Part print with two shaded views. Sizes in mm from the minimum x, y, z corner. A direction names the side the tool comes from. Give positions to 0.01 mm unless a question says otherwise; leave off trailing zeros. Write each loop counter-clockwise with the first axis right and the second up, starting at its lowest first coordinate (ties: lowest second). Pieces come first, ordered by that corner, then holes.
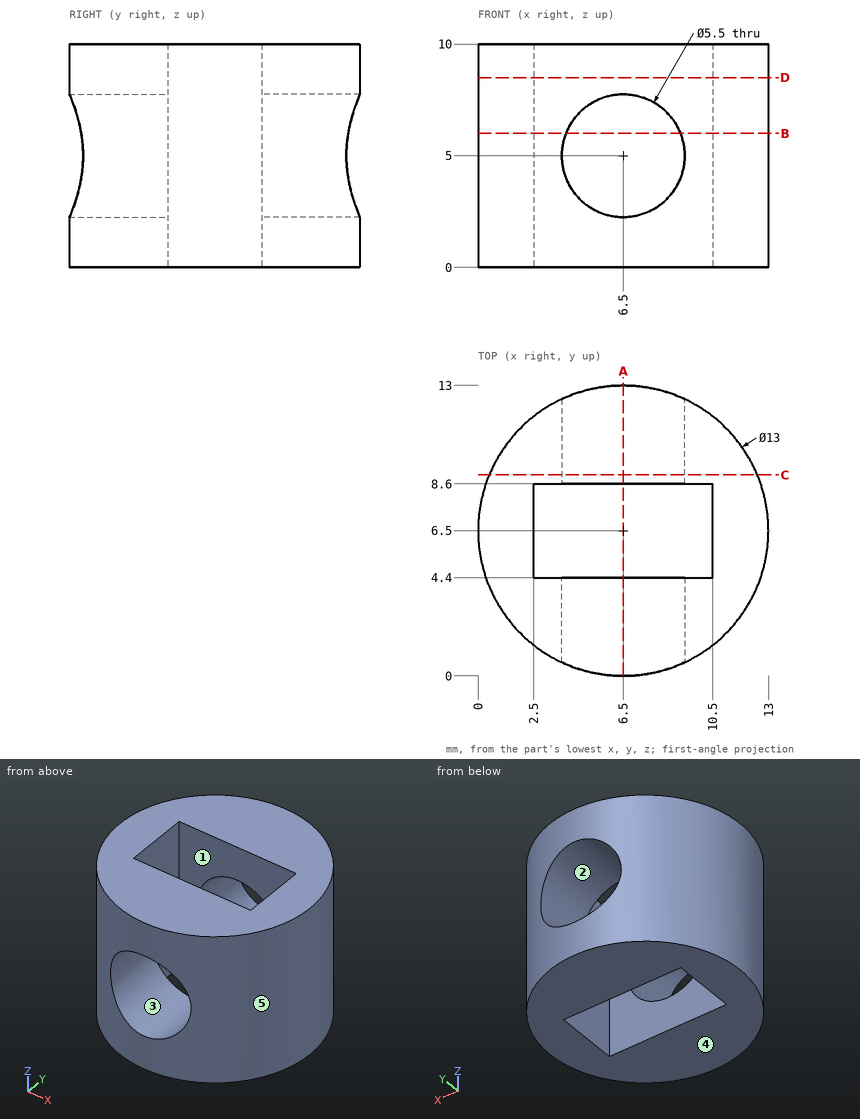
1) Saw through at B-B, the plane z = 6. Write the cut outline in (x, y), then the cut area to 3 significant figures.
Answers follow:
outline: (2.5, 4.4) - (2.5, 8.6) - (3.94, 8.6) - (3.94, 12.47) arc R6.5 ccw to (3.94, 0.53) - (3.94, 4.4) - close; (9.06, 0.53) arc R6.5 ccw to (9.06, 12.47) - (9.06, 8.6) - (10.5, 8.6) - (10.5, 4.4) - (9.06, 4.4) - close
area: 55.8 mm2
2) 3-axis set-ups, long thin cutter, end or side, ignore diameter. For the marked faces 1 and 2: which of +Z, -Z, +X, -X, +Y, -Y reach the whole face in a straight line?
Answers follow:
face 1: +Z, -Z
face 2: +Y, -Y
3) Two-plate mould, pull along X, no slides. Class the marked faces 3, 4 and 5: +X half, -X half, draft (parallel to the pull), parting line (faces both ways), or undercut.
Answers follow:
face 3: undercut
face 4: draft
face 5: parting line
4) Saw through at D-D, the plane z = 8.5. Write the cut outline in (x, y), then the cut area to 3 significant figures.
Answers follow:
outline: circle Ø13 at (6.5, 6.5); hole (2.5, 4.4) - (10.5, 4.4) - (10.5, 8.6) - (2.5, 8.6) - close
area: 99.1 mm2
5) Saw through at A-A, the plane x = 6.5. Write the cut outline in (y, z), then the cut area to 3 significant figures.
Answers follow:
outline: (0, 0) - (4.4, 0) - (4.4, 2.25) - (0, 2.25) - close; (0, 7.75) - (4.4, 7.75) - (4.4, 10) - (0, 10) - close; (8.6, 0) - (13, 0) - (13, 2.25) - (8.6, 2.25) - close; (8.6, 7.75) - (13, 7.75) - (13, 10) - (8.6, 10) - close
area: 39.6 mm2
6) Saw through at C-C, the plane y = 9. Write the cut outline in (x, z), then the cut area to 3 significant figures.
Answers follow:
outline: (0.5, 0) - (12.5, 0) - (12.5, 10) - (0.5, 10) - close; hole circle Ø5.5 at (6.5, 5)
area: 96.2 mm2
7) Pin check, flat tips, straight feed: pin 1 Ø3 at (y, z) = (2, 7.5) entering from -X; pin 2 Ø4 at (x, z) = (6.5, 4.5) entering from +Y; pin 3 Ø2 at (x, z) = (10, 2) entering from +Y. Stop position of each tip, or through.
Answers follow:
pin 1: stops at x = 0.73
pin 2: passes through
pin 3: stops at y = 12.5
8) Wall check: L1, parallel to Z at x = 6.5, y = 1.1; L2, parallel to X at y = 10.5, z = 3; L3, parallel to Y at x = 9.5, z = 5. Give the ranges that are in metal, low to high.
Answers follow:
L1: z = 0 to 2.25, 7.75 to 10
L2: x = 1.38 to 4.61, 8.39 to 11.62
L3: y = 0.73 to 4.4, 8.6 to 12.27
